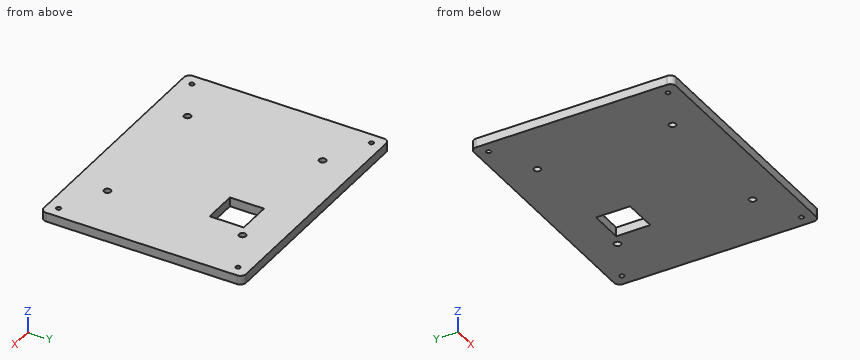
Autodesk Inventor part; units mm, degrees
ref_plane "YZ Plane" through (0, 0, 0) normal (1, 0, 0) x (0, 1, 0)
ref_plane "XZ Plane" through (0, 0, 0) normal (0, 1, 0) x (-1, 0, 0)
ref_plane "XY Plane" through (0, 0, 0) normal (0, 0, 1) x (1, 0, 0)
sketch "Sketch1" plane through (0, 0, 0) normal (0, 0, 1) x (1, 0, 0)
  line L0 (-109, 89) -> (109, 89)
  line L1 (109, 89) -> (109, -89)
  line L2 (109, -89) -> (-109, -89)
  line L3 (-109, -89) -> (-109, 89)
  line L4 (20, 55) -> (50, 55)
  line L5 (50, 55) -> (50, 25)
  line L6 (50, 25) -> (20, 25)
  line L7 (20, 25) -> (20, 55)
  point P0 (0, 0)
  dimension "d0" = 218
  dimension "d1" = 178
  dimension "d2" = 109
  dimension "d3" = 89
  dimension "d4" = 20
  dimension "d5" = 25
  dimension "d6" = 30
  dimension "d7" = 30
extrude "Extrusion1" add sketch "Sketch1" along normal blind 8
fillet "Fillet1" radius 5 4 edges at (-109, -89, 4) (109, -89, 4) (109, 89, 4) (-109, 89, 4)
sketch "Sketch2" plane through (0, 0, 8) normal (0, 0, 1) x (1, 0, 0)
  line L0 (-99, 79) -> (99, 79)
  line L1 (99, 79) -> (99, -79)
  line L2 (99, -79) -> (-99, -79)
  line L3 (-99, -79) -> (-99, 79)
  line L4 (109, -84) -> (109, 84)
  line L5 (104, 89) -> (-104, 89)
  line L6 (-109, 84) -> (-109, -84)
  line L7 (-104, -89) -> (104, -89)
  circle A0 centre (-99, 79) radius 2
  point P0 (0, 0)
  dimension "d11" = 10
  dimension "d12" = 10
  dimension "d13" = 10
  dimension "d14" = 10
  dimension "d15" = 4
hole "Hole1" at (-99, 79, 8) at (99, 79, 8) at (99, -79, 8) at (-99, -79, 8) direction (0, 0, -1) diameter 4 end through all
sketch "Sketch3" plane through (0, 0, 8) normal (0, 0, 1) x (1, 0, 0)
  line L0 (-59.5, 59.5) -> (59.5, 59.5)
  line L1 (59.5, 59.5) -> (59.5, -59.5)
  line L2 (59.5, -59.5) -> (-59.5, -59.5)
  line L3 (-59.5, -59.5) -> (-59.5, 59.5)
  circle A0 centre (-59.5, 59.5) radius 3
  point P0 (0, 0)
  dimension "d23" = 119
  dimension "d24" = 119
  dimension "d25" = 59.5
  dimension "d26" = 59.5
  dimension "d27" = 6
hole "Hole2" at (-59.5, 59.5, 8) at (59.5, 59.5, 8) at (59.5, -59.5, 8) at (-59.5, -59.5, 8) direction (0, 0, -1) diameter 6 end through all
equation "\"d16\" = d15"
equation "\"d28\" = d27"
properties part number "WaagePlexiUnterseite" material "PET Plastic"
The listing builds one solid part. Answer for the finished solid, in the listing's coordinates (mm). Give positions to 0.01 mm unless a question says otherwise; leave off trailing zeros. Order: outer loops, then holes, each group sorted by start corner. A loop starts at its lowest first (then second) coordinate and runs counter-clockwise, first axis right, second up.
Item 1: Given pin 1 Ø3.5 at (x, y) = (99, 79) entering from -Z, flat-ended and moving along its own axis, determine where the tip first touches the part or whether it passes through.
From the geometry:
pin 1: passes through
Item 2: The part is cut by section B-B, the plane y = 30. Give the vertices of the cut face in (x, z).
From the geometry:
outline: (-109, 0) - (20, 0) - (20, 8) - (-109, 8) - close; (50, 0) - (109, 0) - (109, 8) - (50, 8) - close
Item 3: The part is cut by section C-C, the plane y = -59.5. Give the vertices of the cut face in (x, z).
From the geometry:
outline: (-109, 0) - (-62.5, 0) - (-62.5, 8) - (-109, 8) - close; (-56.5, 0) - (56.5, 0) - (56.5, 8) - (-56.5, 8) - close; (62.5, 0) - (109, 0) - (109, 8) - (62.5, 8) - close
Item 4: Find the intervals of material crossed by probe 1 along X at (y, z) = (59.5, 5); probe 2 along X at (y, z) = (79, 5.75); probe 3 along Y at (x, z) = (-99, 4.5), in increasing order.
From the geometry:
probe 1: x = -109 to -62.5, -56.5 to 56.5, 62.5 to 109
probe 2: x = -109 to -101, -97 to 97, 101 to 109
probe 3: y = -89 to -81, -77 to 77, 81 to 89
Item 5: The part is cut by section A-A, the plane x = -59.5. Give the vertices of the cut face in (y, z).
From the geometry:
outline: (-89, 0) - (-62.5, 0) - (-62.5, 8) - (-89, 8) - close; (-56.5, 0) - (56.5, 0) - (56.5, 8) - (-56.5, 8) - close; (62.5, 0) - (89, 0) - (89, 8) - (62.5, 8) - close
